```python
from build123d import *

# Parameters (mm, degrees)
SKETCH7_R           = 15
SKETCH7_R_2         = 2.625
SKETCH7_R_3         = 8
BOSS_EXTRUDE1_DEPTH = 2.5


# Read off the part's stored shape, not the designer's step: 211-0022 (28 Tooth Bevel Gear).STEP<1>
with BuildPart() as part:
    # Sketch7 → Boss-Extrude1 (new body)
    with BuildSketch(Plane.ZY.offset(-1.3887)):
        Circle(SKETCH7_R)
        with Locations((-8, 8)):
            Circle(SKETCH7_R_2, mode=Mode.SUBTRACT)
        with Locations((-11.313708499, 0)):
            Circle(SKETCH7_R_2, mode=Mode.SUBTRACT)
        with Locations((-8, -8)):
            Circle(SKETCH7_R_2, mode=Mode.SUBTRACT)
        with Locations((0, -11.313708499)):
            Circle(SKETCH7_R_2, mode=Mode.SUBTRACT)
        with Locations((8, -8)):
            Circle(SKETCH7_R_2, mode=Mode.SUBTRACT)
        with Locations((11.313708499, 0)):
            Circle(SKETCH7_R_2, mode=Mode.SUBTRACT)
        with Locations((8, 8)):
            Circle(SKETCH7_R_2, mode=Mode.SUBTRACT)
        with Locations((0, 11.313708499)):
            Circle(SKETCH7_R_2, mode=Mode.SUBTRACT)
        Circle(SKETCH7_R_3, mode=Mode.SUBTRACT)
    extrude(amount=BOSS_EXTRUDE1_DEPTH)


solid = part.part
```
Work out the finished part from the listing and answer in its coordinate system (mm). Round coordinates to 2 decimals unless told otherwise and drop trailing zeros. Write each loop counter-clockwise with the first axis right and the second up, starting at its lowest first coordinate (ties: lowest second). Pieces come first, ordered by that corner, then holes. Notation, with made-up numbers: (-6, 55.25) - (41, 55.25) arc R24 cw to (41, 88.25) - close; hole circle Ø8 at (32, 81.5). An arc over 180 degrees is marked (long way). Return JSON: item names as keys, results as strings. Group by question number.
Q1. The part is cut by section A-A on y = 0. Write down the section's boundary in (x, z).
Q2. The part is cut by section D-D on z = -5. Write down the section's boundary in (x, y) (3 decimals).
Q3. Each of these flat-tipped pins is pushed along its axis until it touches: pin 1 Ø1.5 at (x, z) = (-0.5, 7) entering from +Y; pin 2 Ø1.5 at (x, y) = (0.5, 1.5) entering from -Z. Where does it stop, or does it pass through?
Q4. The part is cut by section C-C on y = 4. Write down the section's boundary in (x, z).
Q5. Find the intervals of material crossed by L1, parallel to Y at x = -0.5, z = 0; L2, parallel to Z at x = 0, y = -2; L3, parallel to Z at x = -0.5, y = -1.5, in increasing order.
Q6. The part is cut by section B-B on z = 7. Write down the section's boundary in (x, y), then the cut area to 3 significant figures.
Q7. The mould has two halves that part along Y. Classify faces 1 (the flat face through (-1.111, 8, 2)), 2 (the cylindrical face through (0.156, 8.115, -10.622)), 3 (the cylindrical face through (0.156, 0.66, -14.985)), 4 (the cylindrical face through (0.16, -7.81, -1.73)): released by +Y, released by -Y, zero draft, split by the parting line, or undercut.
Solved:
{
 "1": {"outline": "(-1.11, -15) - (1.39, -15) - (1.39, -13.94) - (-1.11, -13.94) - close; (-1.11, -8.69) - (1.39, -8.69) - (1.39, -8) - (-1.11, -8) - close; (-1.11, 8) - (1.39, 8) - (1.39, 8.69) - (-1.11, 8.69) - close; (-1.11, 13.94) - (1.39, 13.94) - (1.39, 15) - (-1.11, 15) - close"},
 "2": {"outline": "(-1.111, -14.142) - (1.389, -14.142) - (1.389, -6.245) - (-1.111, -6.245) - close; (-1.111, 6.245) - (1.389, 6.245) - (1.389, 14.142) - (-1.111, 14.142) - close"},
 "3": {"pin 1": "y = 13.64", "pin 2": "z = -14.98"},
 "4": {"outline": "(-1.11, -14.46) - (1.39, -14.46) - (1.39, -6.93) - (-1.11, -6.93) - close; (-1.11, 6.93) - (1.39, 6.93) - (1.39, 14.46) - (-1.11, 14.46) - close"},
 "5": {"L1": "-15 to -13.94, -8.69 to -8, 8 to 8.69, 13.94 to 15", "L2": "-14.87 to -13.01, -9.61 to -7.75, 7.75 to 9.61, 13.01 to 14.87", "L3": "-14.92 to -13.47, -9.16 to -7.86, 7.86 to 9.16, 13.47 to 14.92"},
 "6": {"outline": "(-1.11, -13.27) - (1.39, -13.27) - (1.39, -10.43) - (-1.11, -10.43) - close; (-1.11, -5.57) - (1.39, -5.57) - (1.39, -3.87) - (-1.11, -3.87) - close; (-1.11, 3.87) - (1.39, 3.87) - (1.39, 5.57) - (-1.11, 5.57) - close; (-1.11, 10.43) - (1.39, 10.43) - (1.39, 13.27) - (-1.11, 13.27) - close", "area": "22.7 mm²"},
 "7": {"face 1": "zero draft", "face 2": "undercut", "face 3": "split by the parting line", "face 4": "undercut"}
}
